Source: three-view drawing plus pictorial views. Frame: mm from the lowest corner of the part. A direction names the side the tool comes from. Coordinates: 2 decimals unless noted, no trailing zeros. Write each loop counter-clockwise with the first axis right and the second up, starting at its lowest first coordinate (ties: lowest second). Pieces come first, ordered by that corner, then holes. Notation, with made-up numbers: (58.5, 7.5) - (79.5, 7.5) arc R19 ccw to (79.5, 39.5) - close; hole circle Ø8 at (74.5, -12.75). An arc over 180 degrees is marked (long way). One line per item, written item: value.
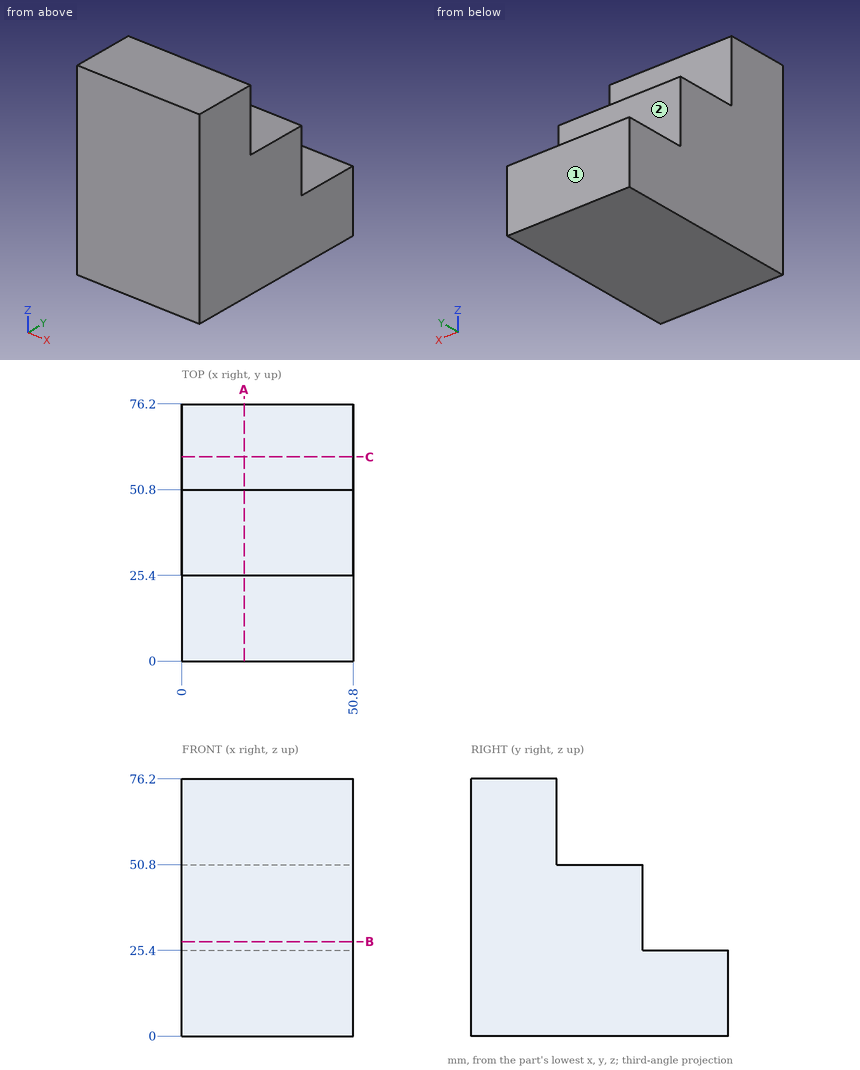
1) Section query C-C on y = 60.5. Output: boundary loops of the cut face in (x, z), then the cut area to 3 significant figures.
Values found:
outline: (0, 0) - (50.8, 0) - (50.8, 25.4) - (0, 25.4) - close
area: 1,290 mm2
2) Section query A-A on x = 18.5. Output: boundary loops of the cut face in (y, z), then the cut area to 3 significant figures.
Values found:
outline: (0, 0) - (76.2, 0) - (76.2, 25.4) - (50.8, 25.4) - (50.8, 50.8) - (25.4, 50.8) - (25.4, 76.2) - (0, 76.2) - close
area: 3,870 mm2
3) Contact query for flat-ended pins moving along their axis: P1, Ø10, axis at x = 45, z = 46, coming from the +Y side; P2, Ø7.5, axis at x = 35, y = 37, coming from the +Z side; P3, Ø7.5, axis at x = 34.5, y = 65.5, coming from the +Z side. Output: stop coordinate, or through.
Values found:
P1: y = 50.8
P2: z = 50.8
P3: z = 25.4
4) Material intervals for line 1 (Z direction, x = 25, y = 73.5); line 2 (Z direction, x = 4, y = 38), sorted ascending.
Values found:
line 1: 0 to 25.4
line 2: 0 to 50.8
5) Section query B-B on z = 28. Output: boundary loops of the cut face in (x, y), then the cut area to 3 significant figures.
Values found:
outline: (0, 0) - (50.8, 0) - (50.8, 50.8) - (0, 50.8) - close
area: 2,580 mm2
6) Reachability of the marked faces 1 and 2 from +Z, -Z, +X, -X, +Y, -Y: full face, straight path, thin tool, end or side. Return the list, or none.
Values found:
face 1: +Z, -Z, +X, -X, +Y
face 2: +Z, +X, -X, +Y
